```python
from build123d import *
from build123d.topology import SkipClean

# Parameters (mm, degrees)
RESSALTO_EXTRUS_O1_DEPTH      = 30
CORTE_EXTRUS_O1_DEPTH         = 54.488316481
CORTE_EXTRUS_O1_DEPTH_BACK    = 54.488316481
ESBO_O3_R                     = 1.1
CORTE_EXTRUS_O6_DEPTH         = 54.488316481
CORTE_EXTRUS_O6_DEPTH_BACK    = 54.488316481
ESBO_O4_W                     = 12
ESBO_O4_H                     = 15
ESBO_O5_R                     = 1.6
CORTE_EXTRUS_O7_DEPTH         = 54.488316481
CORTE_EXTRUS_O9_START         = 1
ESBO_O7_W                     = 15
ESBO_O7_H                     = 15
CORTE_EXTRUS_O9_DEPTH         = 8
CORTE_EXTRUS_O11_REACH        = 55.488
ESBO_O9_R                     = 1.6
ESBO_O8_R                     = 3
CORTE_EXTRUS_O10_DEPTH        = 2
CORTE_EXTRUS_O14_DEPTH        = 43.308391603
CORTE_EXTRUS_O14_DEPTH_BACK   = 2
CORTE_EXTRUS_O16_DEPTH        = 55.626001135
CORTE_EXTRUS_O16_DEPTH_BACK   = 1
ESBO_O15_R                    = 2.1
FILETE1_R                     = 4
ESBO_O16_W                    = 10
ESBO_O16_H                    = 3.82
RESSALTO_EXTRUS_O2_DEPTH      = 2
ESBO_O17_W                    = 15.9
ESBO_O17_H                    = 2.8
RESSALTO_EXTRUS_O3_DEPTH      = 3.5
RESSALTO_EXTRUS_O4_DEPTH      = 6
RESSALTO_EXTRUS_O4_DEPTH_BACK = 1
ESBO_O20_R                    = 3.6
ESBO_O20_R_2                  = 1.6


with BuildPart() as part:
    # Esboço1 → Ressalto-extrusão1 (new body)
    with BuildSketch(Plane.XY):
        with BuildLine():
            Line((0, 0), (3, 0))
            Line((3, 0), (3, 8))
            ThreePointArc((3, 8), (4.464466094, 11.535533906), (8, 13))
            Line((8, 13), (15, 13))
            Line((15, 13), (15, 21))
            Line((15, 21), (-13, 21))
            Line((-13, 21), (-13, 36))
            Line((-13, 36), (1, 36))
            Line((1, 36), (1, 40))
            Line((1, 40), (-19, 40))
            Line((-19, 40), (-19, 17))
            Line((-19, 17), (0, 17))
            Line((0, 17), (0, 0))
        make_face()
    extrude(amount=RESSALTO_EXTRUS_O1_DEPTH)

    # Esboço3 → Corte-extrusão1 (cut, two sides: drawn at the far end of the back side and taken through both)
    with BuildSketch(Plane(origin=(0, 0, 0), x_dir=(0, 0, -1), z_dir=(1, 0, 0)).offset(-CORTE_EXTRUS_O1_DEPTH_BACK)):
        with Locations((-8.5, 14.5)):
            Circle(ESBO_O3_R)
        with Locations(Location((-21.5, 14.5, 0), (0, 0, 90))):
            Circle(ESBO_O3_R)
        with Locations(Location((-8.5, 2.5, 0), (0, 0, 90))):
            Circle(ESBO_O3_R)
        with Locations(Location((-21.5, 2.5, 0), (0, 0, 90))):
            Circle(ESBO_O3_R)
    extrude(amount=CORTE_EXTRUS_O1_DEPTH + CORTE_EXTRUS_O1_DEPTH_BACK, mode=Mode.SUBTRACT)

    # Esboço4 → Corte-extrusão6 (cut, two sides: drawn at the far end of the back side and taken through both)
    with BuildSketch(Plane(origin=(0, 0, 0), x_dir=(1, 0, 0), z_dir=(0, 1, 0)).offset(-CORTE_EXTRUS_O6_DEPTH_BACK)):
        with Locations((9, -22.5)):
            Rectangle(ESBO_O4_W, ESBO_O4_H)
    extrude(amount=CORTE_EXTRUS_O6_DEPTH + CORTE_EXTRUS_O6_DEPTH_BACK, mode=Mode.SUBTRACT)

    # Esboço5 → Corte-extrusão7 (cut, through all)
    with BuildSketch(Plane(origin=(0, 40, 0), x_dir=(1, 0, 0), z_dir=(0, 1, 0))):
        with Locations(Location((-5, -22, 0), (0, 0, 270))):
            Circle(ESBO_O5_R)
        with Locations(Location((-15.7, -11.32, 0), (0, 0, 180))):
            Circle(ESBO_O5_R)
        with Locations(Location((11, -7.5, 0), (0, 0, 180))):
            Circle(ESBO_O5_R)
    extrude(amount=-CORTE_EXTRUS_O7_DEPTH, mode=Mode.SUBTRACT)

    # Esboço7 → Corte-extrusão9 (cut)
    with BuildSketch(Plane(origin=(0, 21, 0), x_dir=(1, 0, 0), z_dir=(0, 1, 0)).offset(CORTE_EXTRUS_O9_START)):
        with Locations((-15.7, -11.32)):
            Rectangle(ESBO_O7_W, ESBO_O7_H)
    extrude(amount=CORTE_EXTRUS_O9_DEPTH, mode=Mode.SUBTRACT)

    # Esboço9 → Corte-extrusão11 (cut, up to next)
    with BuildSketch(Plane(origin=(0, 40, 0), x_dir=(1, 0, 0), z_dir=(0, 1, 0)), mode=Mode.PRIVATE) as corte_extrus_o11_sk1:
        with Locations(Location((-4, -7.5, 0), (0, 0, 180))):
            Circle(ESBO_O9_R)
    corte_extrus_o11_tool1 = extrude(corte_extrus_o11_sk1.sketch, amount=-CORTE_EXTRUS_O11_REACH, mode=Mode.PRIVATE) & part.part
    add(corte_extrus_o11_tool1.solids().sort_by_distance((-4, 40, 7.5))[0], mode=Mode.SUBTRACT)

    # Esboço8 → Corte-extrusão10 (cut)
    with BuildSketch(Plane(origin=(0, 40, 0), x_dir=(1, 0, 0), z_dir=(0, 1, 0))):
        with Locations(Location((-15.7, -11.32, 0), (0, 0, 180))):
            Circle(ESBO_O8_R)
        with Locations(Location((-5, -22, 0), (0, 0, 180))):
            Circle(ESBO_O8_R)
        with Locations(Location((-4, -7.5, 0), (0, 0, 180))):
            Circle(ESBO_O8_R)
    extrude(amount=-CORTE_EXTRUS_O10_DEPTH, mode=Mode.SUBTRACT)

    # Esboço14 → Corte-extrusão14 (cut, two sides: drawn at the far end of the back side and taken through both)
    with BuildSketch(Plane.XZ.offset(-17).offset(-CORTE_EXTRUS_O14_DEPTH_BACK)):
        with BuildLine():
            Line((11, 11), (15, 11))
            Line((15, 11), (15, 4))
            Line((15, 4), (11, 4))
            ThreePointArc((11, 4), (7.5, 7.5), (11, 11))
        make_face()
        Polygon((-5, 25.233161507), (-7.8, 23.616580754), (-7.8, 20.383419246), (-5, 18.766838493), (-2.2, 20.383419246), (-2.2, 23.616580754), align=None)
        Polygon((-15.7, 14.553161507), (-18.5, 12.936580754), (-18.5, 9.703419246), (-15.7, 8.086838493), (-12.9, 9.703419246), (-12.9, 12.936580754), align=None)
    extrude(amount=CORTE_EXTRUS_O14_DEPTH + CORTE_EXTRUS_O14_DEPTH_BACK, mode=Mode.SUBTRACT)

    # Esboço15 → Corte-extrusão16 (cut, two sides: drawn at the far end of the back side and taken through both)
    with BuildSketch(Plane(origin=(3, 0, 0), x_dir=(0, 0, -1), z_dir=(1, 0, 0)).offset(-CORTE_EXTRUS_O16_DEPTH_BACK)):
        with Locations(Location((-21.5, 14.5, 0), (0, 0, 90))):
            Circle(ESBO_O15_R)
        with Locations(Location((-8.5, 14.5, 0), (0, 0, 313.540252108))):
            Circle(ESBO_O15_R)
        with Locations(Location((-8.5, 2.5, 0), (0, 0, 90))):
            Circle(ESBO_O15_R)
        with Locations(Location((-21.5, 2.5, 0), (0, 0, 90))):
            Circle(ESBO_O15_R)
    extrude(amount=CORTE_EXTRUS_O16_DEPTH + CORTE_EXTRUS_O16_DEPTH_BACK, mode=Mode.SUBTRACT)

    # Filete1
    # the kernel refuses this fillet: 4 mm, written as the material it adds along each edge
    with BuildSketch(Plane(origin=(-13, 21, 0), x_dir=(1, 0, 0), z_dir=(0, 0, 1))) as filete1_piece_1_section:
        with BuildLine():
            CenterArc((FILETE1_R, FILETE1_R), FILETE1_R, 180, 90)
            Line((0, FILETE1_R), (0, 0))
            Line((0, 0), (FILETE1_R, 0))
        make_face()
    filete1_piece_1 = extrude(amount=30, mode=Mode.PRIVATE)
    filete1_piece_1 = split(filete1_piece_1, bisect_by=Plane(origin=(-11.759467995, 21.365337359, 3.82), z_dir=(0, 0, -1)), keep=Keep.TOP, mode=Mode.PRIVATE)
    filete1_piece_1 = split(filete1_piece_1, bisect_by=Plane(origin=(-11.759467995, 22, 1.91), z_dir=(0, -1, 0)), keep=Keep.TOP, mode=Mode.PRIVATE)
    add(filete1_piece_1)
    with BuildSketch(Plane(origin=(-13, 21, 0), x_dir=(1, 0, 0), z_dir=(0, 0, 1))) as filete1_piece_2_section:
        with BuildLine():
            CenterArc((FILETE1_R, FILETE1_R), FILETE1_R, 180, 90)
            Line((0, FILETE1_R), (0, 0))
            Line((0, 0), (FILETE1_R, 0))
        make_face()
    filete1_piece_2 = extrude(amount=30, mode=Mode.PRIVATE)
    filete1_piece_2 = split(filete1_piece_2, bisect_by=Plane(origin=(-12.678584174, 22.84777915, 3.82), z_dir=(0, 0, -1)), keep=Keep.TOP, mode=Mode.PRIVATE)
    filete1_piece_2 = split(filete1_piece_2, bisect_by=Plane(origin=(-12.678584174, 22, 1.91), z_dir=(0, 1, 0)), keep=Keep.TOP, mode=Mode.PRIVATE)
    add(filete1_piece_2)
    with BuildSketch(Plane(origin=(-13, 21, 0), x_dir=(1, 0, 0), z_dir=(0, 0, 1))) as filete1_piece_3_section:
        with BuildLine():
            CenterArc((FILETE1_R, FILETE1_R), FILETE1_R, 180, 90)
            Line((0, FILETE1_R), (0, 0))
            Line((0, 0), (FILETE1_R, 0))
        make_face()
    filete1_piece_3 = extrude(amount=30, mode=Mode.PRIVATE)
    filete1_piece_3 = split(filete1_piece_3, bisect_by=Plane(origin=(-11.759467995, 21.365337359, 3.82), z_dir=(0, 0, 1)), keep=Keep.TOP, mode=Mode.PRIVATE)
    filete1_piece_3 = split(filete1_piece_3, bisect_by=Plane(origin=(-11.759467995, 22, 11.32), z_dir=(0, -1, 0)), keep=Keep.TOP, mode=Mode.PRIVATE)
    filete1_piece_3 = split(filete1_piece_3, bisect_by=Plane(origin=(-11.759467995, 21.365337359, 18.82), z_dir=(0, 0, -1)), keep=Keep.TOP, mode=Mode.PRIVATE)
    add(filete1_piece_3)
    with BuildSketch(Plane(origin=(-13, 21, 0), x_dir=(1, 0, 0), z_dir=(0, 0, 1))) as filete1_piece_4_section:
        with BuildLine():
            CenterArc((FILETE1_R, FILETE1_R), FILETE1_R, 180, 90)
            Line((0, FILETE1_R), (0, 0))
            Line((0, 0), (FILETE1_R, 0))
        make_face()
    filete1_piece_4 = extrude(amount=30, mode=Mode.PRIVATE)
    filete1_piece_4 = split(filete1_piece_4, bisect_by=Plane(origin=(-11.759467995, 22, 24.41), z_dir=(0, -1, 0)), keep=Keep.TOP, mode=Mode.PRIVATE)
    filete1_piece_4 = split(filete1_piece_4, bisect_by=Plane(origin=(-11.759467995, 21.365337359, 18.82), z_dir=(0, 0, 1)), keep=Keep.TOP, mode=Mode.PRIVATE)
    add(filete1_piece_4)
    with BuildSketch(Plane(origin=(-13, 21, 0), x_dir=(1, 0, 0), z_dir=(0, 0, 1))) as filete1_piece_5_section:
        with BuildLine():
            CenterArc((FILETE1_R, FILETE1_R), FILETE1_R, 180, 90)
            Line((0, FILETE1_R), (0, 0))
            Line((0, 0), (FILETE1_R, 0))
        make_face()
    filete1_piece_5 = extrude(amount=30, mode=Mode.PRIVATE)
    filete1_piece_5 = split(filete1_piece_5, bisect_by=Plane(origin=(-12.678584174, 22, 24.41), z_dir=(0, 1, 0)), keep=Keep.TOP, mode=Mode.PRIVATE)
    filete1_piece_5 = split(filete1_piece_5, bisect_by=Plane(origin=(-12.678584174, 22.84777915, 18.82), z_dir=(0, 0, 1)), keep=Keep.TOP, mode=Mode.PRIVATE)
    add(filete1_piece_5)
    with BuildSketch(Plane(origin=(-13, 36, 0), x_dir=(1, 0, 0), z_dir=(0, 0, 1))) as filete1_piece_6:
        with BuildLine():
            CenterArc((FILETE1_R, -FILETE1_R), FILETE1_R, 90, 90)
            Line((0, -FILETE1_R), (0, 0))
            Line((0, 0), (FILETE1_R, 0))
        make_face()
    extrude(amount=30)
    # the kernel refuses this fillet: 4 mm, written as the material it takes off along each edge
    with BuildSketch(Plane(origin=(-10, 0, 0), x_dir=(0, 0, 1), z_dir=(1, 0, 0))) as filete1_2_piece_1:
        with BuildLine():
            CenterArc((FILETE1_R, -FILETE1_R), FILETE1_R, 90, 90)
            Line((0, -FILETE1_R), (0, 0))
            Line((0, 0), (FILETE1_R, 0))
        make_face()
    extrude(amount=23, mode=Mode.SUBTRACT)
    with BuildSketch(Plane(origin=(-10, 0, 30), x_dir=(0, 0, -1), z_dir=(1, 0, 0))) as filete1_2_piece_2:
        with BuildLine():
            CenterArc((FILETE1_R, FILETE1_R), FILETE1_R, 180, 90)
            Line((0, FILETE1_R), (0, 0))
            Line((0, 0), (FILETE1_R, 0))
        make_face()
    extrude(amount=23, mode=Mode.SUBTRACT)
    with BuildSketch(Plane(origin=(3, 21, 15), x_dir=(-1, 0, 0), z_dir=(0, 0, 1))) as filete1_2_piece_3:
        with BuildLine():
            CenterArc((FILETE1_R, FILETE1_R), FILETE1_R, 180, 90)
            Line((0, FILETE1_R), (0, 0))
            Line((0, 0), (FILETE1_R, 0))
        make_face()
    extrude(amount=25, mode=Mode.SUBTRACT)
    with BuildSketch(Plane(origin=(1, 26, 0), x_dir=(0, 0, 1), z_dir=(0, 1, 0)), Plane(origin=(15, 13, -10), x_dir=(-1, 0, 0), z_dir=(0, 0, 1)), Plane(origin=(15, 13, 1), x_dir=(-1, 0, 0), z_dir=(0, 0, 1)), Plane(origin=(1, 26, 30), x_dir=(-1, 0, 0), z_dir=(0, 1, 0))) as filete1_2_piece_4:
        with BuildLine():
            CenterArc((FILETE1_R, -FILETE1_R), FILETE1_R, 90, 90)
            Line((0, -FILETE1_R), (0, 0))
            Line((0, 0), (FILETE1_R, 0))
        make_face()
    extrude(amount=24, mode=Mode.SUBTRACT)

    # Esboço16 → Ressalto-extrusão2 (add)
    with BuildSketch(Plane(origin=(0, 21, 0), x_dir=(1, 0, 0), z_dir=(0, 1, 0))):
        with Locations((-14, -1.91)):
            Rectangle(ESBO_O16_W, ESBO_O16_H)
    extrude(amount=RESSALTO_EXTRUS_O2_DEPTH)

    # Esboço17 → Ressalto-extrusão3 (add)
    with BuildSketch(Plane(origin=(0, 21, 0), x_dir=(1, 0, 0), z_dir=(0, 1, 0))):
        with Locations((-1.05, -7.5)):
            Rectangle(ESBO_O17_W, ESBO_O17_H)
    extrude(amount=RESSALTO_EXTRUS_O3_DEPTH)

    # Esboço20 → Ressalto-extrusão4 (add, two sides: drawn at the far end of the back side and taken through both)
    with SkipClean():  # the faces are left unmerged after this step: merging them gives an invalid solid
        with BuildSketch(Plane(origin=(0, 21, 0), x_dir=(1, 0, 0), z_dir=(0, 1, 0)).offset(-RESSALTO_EXTRUS_O4_DEPTH_BACK)):
            with Locations((-5, -22)):
                Circle(ESBO_O20_R)
            with Locations(Location((-5, -22, 0), (0, 0, 180))):
                Circle(ESBO_O20_R_2, mode=Mode.SUBTRACT)
        extrude(amount=RESSALTO_EXTRUS_O4_DEPTH + RESSALTO_EXTRUS_O4_DEPTH_BACK)


solid = part.part
```
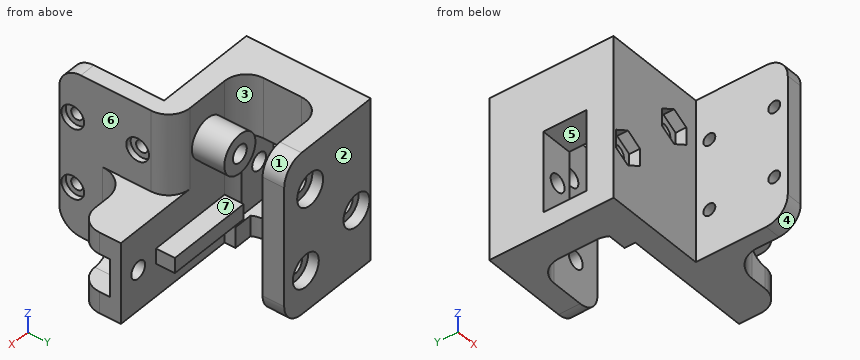
Verification items for the finished model (mm, model axes). Face numbers are marked on the shaded views. A direction names the side the tool comes from. Coordinates: 2 decimals unless noted, no trailing zeros. Order: outer loops, then holes, each group sorted by start corner. A loop starts at its lowest first (then second) coordinate and runs counter-clockwise, first axis right, second up. Notation, with made-up numbers: (14, -2) - (40, -2) arc R32 cw to (40, 26) - close; hole circle Ø3 at (-8, 8). An arc over 180 degrees is marked (long way). Return JSON: item names as keys, results as strings.
(1) Mould release check, pull along Y, two halves, no side actions. Record for the marked faces 1, 2, 3 and 4: pulls with the +Y half, pulls with the -Y half, needs draft (parallel to the pull), parting line crosses it, or undercut.
Filled sheet:
{"face 1": "needs draft", "face 2": "pulls with the +Y half", "face 3": "undercut", "face 4": "pulls with the -Y half"}
(2) Section check B-B, the plane y = 14.5. Record the cut outline in (x, z), and give its area (3 significant figures).
Filled sheet:
{"outline": "(0, 0) - (14.12, 0) - (14.12, 4) - (11, 4) arc R3.5 cw to (7.68, 6.4) - (2, 6.4) - (2, 7.4) - (0, 7.4) - close; (0, 9.6) - (2, 9.6) - (2, 10.6) - (9.38, 10.6) arc R3.5 cw to (11, 11) - (14.12, 11) - (14.12, 15) - (3, 15) - (3, 19.4) - (2, 19.4) - (2, 20.4) - (0, 20.4) - close; (0, 22.6) - (2, 22.6) - (2, 23.6) - (3, 23.6) - (3, 30) - (0, 30) - close", "area": "178 mm^2"}
(3) Access from +Z, -Z, +X, -X, +Y, -Y to the whole of each face (thin tool, end or side, straight path). Record for the marked faces 5, 6 and 7.
Filled sheet:
{"face 5": "-X", "face 6": "+Z, +X, -Y", "face 7": "+X"}
(4) Thickness scan on line 1 along Y through (x, z) = (1.3, 8.5); line 2 along Y through (x, z) = (-1.5, 16); line 3 along Y through (x, z) = (-6.5, 9). Record the ranges inside material, lowest first.
Filled sheet:
{"line 1": "y = 0 to 1.4, 3.6 to 13.4, 15.6 to 24.5", "line 2": "y = 17 to 21, 36 to 40", "line 3": "y = 17 to 21, 36 to 38"}
(5) Section check D-D, the plane z = 2. Record the cut outline in (x, y), and give its area (3 significant figures).
Filled sheet:
{"outline": "(-19, 17) - (0, 17) - (0, 0.54) - (3, 0.54) - (3, 8) arc R5 cw to (8, 13) - (11, 13) arc R4 ccw to (15, 17) - (15, 21) - (-9, 21) - (-9, 23) - (-12.46, 23) arc R4 cw to (-13, 25) - (-13, 32) arc R4 cw to (-9, 36) - (0.46, 36) - (0.46, 40) - (-19, 40) - close", "area": "415 mm^2"}
(6) Go/stop test with flat-tipped pins: pin 1 (2 mm diameter, centred on y = 14.5, z = 21.5, fed in from -X); pin 2 (8 mm diameter, centred on x = -9.5, z = 25, fed in from -Y); pin 3 (10 mm diameter, centred on y = 11.5, z = 8.5, fed in from -X); pin 4 (4.5 mm diameter, centred on y = 37.5, z = 14, fed in from +X). Record where each tip stops, or that it passes through.
Filled sheet:
{"pin 1": "passes through", "pin 2": "stops at y = 17", "pin 3": "stops at x = 0", "pin 4": "stops at x = 1"}
(7) Section check A-A, the plane y = 37. Record the cut outline in (x, z).
Filled sheet:
{"outline": "(-19, 0) - (-3, 0) arc R4 ccw to (1, 4) - (1, 26) arc R4 ccw to (-3, 30) - (-19, 30) - close; hole circle Ø3.2 at (-15.7, 11.32); hole circle Ø3.2 at (-5, 22); hole circle Ø3.2 at (-4, 7.5)"}
(8) Section check C-C, the plane x = -11. Record the cut outline in (y, z).
Filled sheet:
{"outline": "(17, 0) - (23, 0) - (23, 3.82) - (21.54, 3.82) - (21.54, 30) - (17, 30) - close; (35.46, 0) - (40, 0) - (40, 30) - (35.46, 30) - close"}
